from build123d import *

# Parameters (mm, degrees)
SKETCH_1_W           = 40.24
SKETCH_1_H           = 26.05
EXTRUDE_1_DEPTH      = 1.6
EXTRUDE_2_DEPTH      = 15.2
EXTRUDE_3_DEPTH      = 4
EXTRUDE_3_DEPTH_BACK = 2


with BuildPart() as part:
    # 草图1 → 凸台-拉伸1 (new body)
    with BuildSketch(Plane(origin=(0, 0, 0), x_dir=(1, 0, 0), z_dir=(0, 1, 0))):
        with Locations((20.12, 13.025)):
            Rectangle(SKETCH_1_W, SKETCH_1_H)
    extrude(amount=EXTRUDE_1_DEPTH)

    # 草图2 → 凸台-拉伸2 (add)
    with BuildSketch(Plane(origin=(0, 1.6, 0), x_dir=(1, 0, 0), z_dir=(0, 1, 0))):
        with BuildLine():
            Line((15.24, 13.025), (25.24, 13.025))
            Line((25.24, 13.025), (35.24, 13.025))
            ThreePointArc((35.24, 13.025), (25.24, 23.025), (15.24, 13.025))
        make_face()
        with BuildLine():
            Line((35.24, 13.025), (25.24, 13.025))
            Line((25.24, 13.025), (15.24, 13.025))
            ThreePointArc((15.24, 13.025), (25.24, 3.025), (35.24, 13.025))
        make_face()
    extrude(amount=EXTRUDE_2_DEPTH)

    # 草图3 → 凸台-拉伸3 (add, two sides)
    with BuildSketch(Plane.ZY) as extrude_3_sk:
        Polygon((-19.275, 7.35), (-19.275, 1.6), (-13.025, 1.6), (-6.775, 1.6), (-6.775, 7.35), align=None)
    extrude(amount=EXTRUDE_3_DEPTH)
    extrude(extrude_3_sk.sketch, amount=-EXTRUDE_3_DEPTH_BACK)


solid = part.part
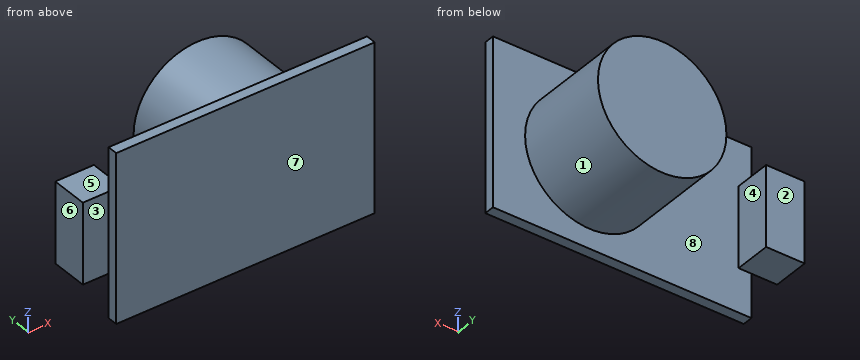
The listing builds one solid part. Answer for the finished solid, in the listing's coordinates (mm). Face numbers are marked on the shaded views. A direction names the side the tool comes from. Round coordinates to 2 decimals unless told otherwise and drop trailing zeros. Write each loop counter-clockwise with the first axis right and the second up, starting at its lowest first coordinate (ties: lowest second). Pieces come first, ordered by that corner, then holes. Notation, with made-up numbers: (50.5, 83.25) - (58.5, 83.25) arc R18 cw to (58.5, 90.25) - close; hole circle Ø8 at (-11, 48). An arc over 180 degrees is marked (long way). Use a Markdown table: item, result. Add a question column.
1. The part is cut by section B-B (z = -18.75). Write down the section's boundary in (x, y).
2. A tool of negligible diameter and unlimited length cuts with its end or side. For the marked faces 1, 2, 3, 4 and 5, from which of +Z, -Z, +X, -X, +Y, -Y can it reach the whole face along a straight path? Write none if from no direction.
3. The part is cut by section C-C (y = 5.25). Write down the section's boundary in (x, z) (3 decimals).
4. Flat-ended cylindrical pins translate along their axes: P1, Ø2, axis at x = -2.5, z = -10, coming from the -Y side; P2, Ø10, axis at y = 7, z = -9, coming from the +X side; P3, Ø5, axis at x = 5.5, z = -10.5, coming from the +Y side. Find the tip coordinate at first contact, or state that the pin passes through.
5. The part is cut by section A-A (x = 25.24). Write down the section's boundary in (y, z) (3 decimals), and give its area (3 significant figures).
6. The part is cut by section D-D (z = -9.75). Write down the section's boundary in (x, y).
7. Consider line 1 (Y direction, x = 34.5, z = -4.5); line 2 (X direction, y = 2.75, z = -14.25); line 3 (X direction, y = 9, z = -12.75). Determine where each line is inside the solid, lowest interval first.
8. For a pull along X with two mould halves and no side action, classify the marked faces 6, 7 and 8 as +X half, -X half, draft (parallel to the pull), parting line (faces both ways), or undercut.
Reported:
| question | item | result |
|---|---|---|
| 1 | outline | (-4, 1.6) - (0, 1.6) - (0, 0) - (40.24, 0) - (40.24, 1.6) - (33.44, 1.6) - (33.44, 16.8) - (17.04, 16.8) - (17.04, 1.6) - (2, 1.6) - (2, 7.35) - (-4, 7.35) - close |
| 2 | face 1 | +Y |
| 2 | face 2 | +Z, -Z, -X, +Y |
| 2 | face 3 | +Z, -Z, -X, -Y |
| 2 | face 4 | +Z, -Z, +Y |
| 2 | face 5 | +Z, -X, +Y |
| 3 | outline | (-4, -19.275) - (2, -19.275) - (2, -6.775) - (-4, -6.775) - close; circle Ø20 at (25.24, -13.025) |
| 4 | P1 | y = 1.6 |
| 4 | P2 | x = 35.24 |
| 4 | P3 | y = 1.6 |
| 5 | outline | (0, -26.05) - (1.6, -26.05) - (1.6, -23.025) - (16.8, -23.025) - (16.8, -3.025) - (1.6, -3.025) - (1.6, 0) - (0, 0) - close |
| 5 | area | 346 mm^2 |
| 6 | outline | (-4, 1.6) - (0, 1.6) - (0, 0) - (40.24, 0) - (40.24, 1.6) - (34.69, 1.6) - (34.69, 16.8) - (15.79, 16.8) - (15.79, 1.6) - (2, 1.6) - (2, 7.35) - (-4, 7.35) - close |
| 7 | line 1 | 0 to 1.6 |
| 7 | line 2 | -4 to 2, 15.32 to 35.16 |
| 7 | line 3 | 15.24 to 35.24 |
| 8 | face 6 | -X half |
| 8 | face 7 | draft |
| 8 | face 8 | undercut |
